Geometry: final body of the model. Coordinates: model frame, mm. A direction names the side the tool comes from. Give positions to 0.01 mm unless a question says otherwise; leave off trailing zeros. Loops run counter-clockwise (first coordinate to the right, second up) from the corner with the lowest first, then second, coordinate; pieces in that order, holes last. Notation, with made-up numbers: (-31.5, 24) -> (-25.5, 24) arc R15 cw to (-25.5, 46) -> close; hole circle Ø5 at (9.25, 86.5). An arc over 180 degrees is marked (long way). Answer in a Markdown table with one row per item. Add a question column.
1) Section query B-B (x = 83.5). Return the cut outline in (y, z), plus the area to 3 significant figures.
2) Section query A-A (z = 6.75). Return the cut outline in (x, y), plus the area to 3 significant figures.
3) Section query C-C (y = 0). Return the cut outline in (x, z).
4) Access query for faces 1 (the flat face through (8, 5.164, 17)), 2 (the flat face through (59, 0, 17)), 3 (the flat face through (8, -5.164, 17)). Directions: +Z, -Z, +X, -X, +Y, -Y. A direction counts if a zero-diameter tool reaches every point of the face in a straight line with its end or side. Return the directions, or none.
5) Section query D-D (x = 16.5). Return the cut outline in (y, z), plus the area to 3 significant figures.
6) First-contact query: P1, Ø7, axis at x = 10.5, z = 16.5, coming from the +Y side; P2, Ø4, axis at x = -67, y = -5, coming from the +Z side; P3, Ø11.5, axis at y = -2.5, z = 16.5, coming from the +X side; P4, Ø5, axis at x = -62, y = 0, coming from the -Z side. Flat tips, straight axial feed; report the tip coordinate or a pass-through.
7) Line query: line 1 (Y direction, x = -62, z = 6); line 2 (Z direction, x = 99.5, y = -9); line 3 (X direction, y = 2, z = 6). Output: solid intervals per line, ascending. Write a range as from..to.
```python
from build123d import *

# Parameters (mm, degrees)
SKETCH_1_W          = 240
SKETCH_1_H          = 46
EXTRUDE_1_DEPTH     = 10
CUT_EXTRUDE_1_DEPTH = 10
SKETCH_3_W          = 66.746798051
SKETCH_3_H          = 10
EXTRUDE_3_DEPTH     = 14
SKETCH_5_R          = 12.5
CUT_EXTRUDE_2_DEPTH = 14
SKETCH_6_R          = 4
CUT_EXTRUDE_3_DEPTH = 10
SKETCH_7_W          = 66.746798051
SKETCH_7_H          = 14
CUT_EXTRUDE_4_DEPTH = 10
SKETCH_8_W          = 100
SKETCH_8_H          = 10.327994094
EXTRUDE_4_DEPTH     = 14
SKETCH_9_R          = 12.5
SKETCH_9_R_2        = 4
EXTRUDE_5_DEPTH     = 10


with BuildPart() as part:
    # 草图1 → 凸台-拉伸1 (new body)
    with BuildSketch(Plane.XY):
        Rectangle(SKETCH_1_W, SKETCH_1_H)
    extrude(amount=EXTRUDE_1_DEPTH)

    # 草图2 → 切除-拉伸1 (cut)
    with BuildSketch(Plane.XY.offset(10)):
        Polygon((-55, 23), (-20.454545455, 21), (40, 21), (40, 17.5), (80, 23), align=None)
        Polygon((80, -23), (40, -17.5), (40, -21), (-20.454545455, -21), (-55, -23), align=None)
        Polygon((40, -21), (40, -17.5), (-20.454545455, -21), align=None)
        Polygon((40, 21), (-20.454545455, 21), (40, 17.5), align=None)
    extrude(amount=-CUT_EXTRUDE_1_DEPTH, mode=Mode.SUBTRACT)

    # 草图3 → 凸台-拉伸3 (add)
    with BuildSketch(Plane.XY.offset(10)):
        with Locations((-11.626600974, 0)):
            Rectangle(SKETCH_3_W, SKETCH_3_H)
    extrude(amount=EXTRUDE_3_DEPTH)

    # 草图5 → 切除-拉伸2 (cut)
    with BuildSketch(Plane.XY.offset(10)):
        with Locations((83.5, 0)):
            Circle(SKETCH_5_R)
    extrude(amount=-CUT_EXTRUDE_2_DEPTH, mode=Mode.SUBTRACT)

    # 草图6 → 切除-拉伸3 (cut)
    with BuildSketch(Plane.XY.offset(10)):
        with Locations((-62, 0)):
            Circle(SKETCH_6_R)
    extrude(amount=-CUT_EXTRUDE_3_DEPTH, mode=Mode.SUBTRACT)

    # 草图7 → 切除-拉伸4 (cut)
    with BuildSketch(Plane.XZ.offset(5)):
        with Locations((-11.626600974, 17)):
            Rectangle(SKETCH_7_W, SKETCH_7_H)
    extrude(amount=-CUT_EXTRUDE_4_DEPTH, mode=Mode.SUBTRACT)

    # 草图8 → 凸台-拉伸4 (add)
    with BuildSketch(Plane.XY.offset(10)):
        with Locations((9, 0)):
            Rectangle(SKETCH_8_W, SKETCH_8_H)
    extrude(amount=EXTRUDE_4_DEPTH)

    # 草图9 → 凸台-拉伸5 (add)
    with BuildSketch(Plane.XY.offset(10)):
        with Locations((83.5, 0)):
            Circle(SKETCH_9_R)
        with Locations((83.5, 0)):
            Circle(SKETCH_9_R_2, mode=Mode.SUBTRACT)
    extrude(amount=-EXTRUDE_5_DEPTH)


solid = part.part
```
Evaluation:
| question | item | result |
|---|---|---|
| 1 | outline | (-23, 0) -> (-4, 0) -> (-4, 10) -> (-23, 10) -> close; (4, 0) -> (23, 0) -> (23, 10) -> (4, 10) -> close |
| 1 | area | 380 mm² |
| 2 | outline | (-120, -23) -> (-55, -23) -> (40, -17.5) -> (80, -23) -> (120, -23) -> (120, 23) -> (80, 23) -> (40, 17.5) -> (-55, 23) -> (-120, 23) -> close; hole circle Ø8 at (-62, 0); hole circle Ø8 at (83.5, 0) |
| 2 | area | 10,200 mm² |
| 3 | outline | (-120, 0) -> (-66, 0) -> (-66, 10) -> (-120, 10) -> close; (-58, 0) -> (79.5, 0) -> (79.5, 10) -> (59, 10) -> (59, 24) -> (-41, 24) -> (-41, 10) -> (-58, 10) -> close; (87.5, 0) -> (120, 0) -> (120, 10) -> (87.5, 10) -> close |
| 4 | face 1 | +Z, +X, -X, +Y |
| 4 | face 2 | +Z, +X, +Y, -Y |
| 4 | face 3 | +Z, +X, -X, -Y |
| 5 | outline | (-18.86, 0) -> (18.86, 0) -> (18.86, 10) -> (5.16, 10) -> (5.16, 24) -> (-5.16, 24) -> (-5.16, 10) -> (-18.86, 10) -> close |
| 5 | area | 522 mm² |
| 6 | P1 | y = 5.16 |
| 6 | P2 | z = 10 |
| 6 | P3 | x = 59 |
| 6 | P4 | through |
| 7 | line 1 | -23..-4, 4..23 |
| 7 | line 2 | 0..10 |
| 7 | line 3 | -120..-65.46, -58.54..80.04, 86.96..120 |
